Autodesk Inventor part; units mm, degrees
ref_plane "YZ Plane" through (0, 0, 0) normal (1, 0, 0) x (0, 1, 0)
ref_plane "XZ Plane" through (0, 0, 0) normal (0, 1, 0) x (-1, 0, 0)
ref_plane "XY Plane" through (0, 0, 0) normal (0, 0, 1) x (1, 0, 0)
sketch "Sketch2" plane through (0, 0, 0) normal (0, 0, 1) x (1, 0, 0)
  line L0 (0, 0) -> (76.2, 0)
  line L1 (76.2, 0) -> (76.2, 50.8)
  line L2 (76.2, 50.8) -> (0, 50.8)
  line L3 (0, 50.8) -> (0, 0)
  line L4 (-25.4, 0) -> (127, 0)
  line L5 (127, 0) -> (127, -50.8)
  line L6 (127, -50.8) -> (-25.4, -50.8)
  line L7 (-25.4, -50.8) -> (-25.4, 0)
  circle A0 centre (-19.05, -6.35) radius 3.175
  circle A1 centre (76.2, -44.45) radius 3.175
  line L8 (-17.8708, -3.4021) -> (77.3792, -41.5021)
  line L9 (-20.2292, -9.2979) -> (75.0208, -47.3979)
  circle A2 centre (25.4, -6.35) radius 3.175
  circle A3 centre (120.65, -44.45) radius 3.175
  line L10 (26.5792, -3.4021) -> (121.8292, -41.5021)
  line L11 (24.2208, -9.2979) -> (119.4708, -47.3979)
  dimension "d0" = 76.2
  dimension "d1" = 50.8
  dimension "d2" = 152.4
  dimension "d3" = 50.8
  dimension "d4" = 25.4
  dimension "d5" = 6.35
  dimension "d6" = 6.35
  dimension "d7" = 6.35
  dimension "d8" = 6.35
  dimension "d9" = 6.35
  dimension "d10" = 6.35
  dimension "d11" = 6.35
  dimension "d12" = 6.35
extrude "Extrusion1" add sketch "Sketch2" along normal blind 6.35
chamfer "Chamfer1" distance 6.35 angle 45 1 edges at (38.1, 50.8, 6.35)
properties part number "Short Wall Lift"
Here's how the part is built. I have some questions about the finished solid (model axes, mm). A direction names the side the tool comes from. Give positions to 0.01 mm unless a question says otherwise; leave off trailing zeros. Order: outer loops, then holes, each group sorted by start corner. A loop starts at its lowest first (then second) coordinate and runs counter-clockwise, first axis right, second up. Notation, with made-up numbers: M 31.25,12 L 78.25,12 A21 cw 78.25,37 Z; hole C 78.25,27.25 d4. An arc over 180 degrees is marked long. Answer as a JSON object with one key per item and string values. Group by question number.
1) We'd pull the mould along Y, two halves only. Please class faces 1 (the flat face through (52, -50.8, 3)), 2 (the flat face through (73.537, -22.185, 3.131)), 3 (the flat face through (127, -25, 3)), 4 (the cylindrical face through (123.623, -45.564, 3.131)): pulls with the +Y half, pulls with the -Y half, needs draft (parallel to the pull), parting line crosses it, or undercut.
2) On a 3-axis mill with a long thin cutter (end or side, diameter ignored), from which of +Z, -Z, +X, -X, +Y, -Y can I reach the whole of each face in a straight line? I mean faces 5 (the flat face through (37.6, 47.6, 3.2)), 6 (the flat face through (101, 0, 3)), 7 (the flat face through (29.087, -22.185, 3.131)), 8 (the flat face through (0, 26, 3)), 9 (the flat face through (50, -11, 0)). Say none if no direction works.
3) Suppose I cut it at C-C, the plane z = 4.5. Count the separate pieces of the cut face and the enclosed holes in it, plus the area to 3 significant figures.
4) Please list where these lines run through material, in increasing order: L1, parallel to Y at x = 54.5, z = 2.5; L2, parallel to Y at x = 38, z = 5.75; L3, parallel to X at y = 8, z = 1.5. Write a range as [from, to].
5) Suppose I cut it at B-B, the plane y = -17. Write out the boundary of the cut face in (x, z), plus the area to 3 significant figures.
6) I'm going to push flat-ended pins straight in: pin 1 Ø3 at (x, z) = (77.5, 2.5) entering from +Y; pin 2 Ø8 at (x, y) = (9.5, 29.5) entering from -Z; pin 3 Ø3 at (y, z) = (21.5, 3) entering from +X. Where does each tip first touch, or does it pass through?
Results found:
{
 "1": {"face 1": "pulls with the -Y half", "face 2": "undercut", "face 3": "needs draft", "face 4": "undercut"},
 "2": {"face 5": "+Z, +X, -X, +Y", "face 6": "+Z, -Z, +X, +Y", "face 7": "+Z, -Z", "face 8": "+Z, -Z, -X, +Y", "face 9": "-Z, +X, -X, +Y, -Y"},
 "3": {"separate pieces": "1", "enclosed holes": "2", "area": "9,900 mm²"},
 "4": {"L1": "[-50.8, -39.19], [-32.35, -21.41], [-14.57, 48.3]", "L2": "[-50.8, -32.59], [-25.75, -14.81], [-7.97, 45.05]", "L3": "[0, 76.2]"},
 "5": {"outline": "M -25.4,0 L -0.97,0 L -0.97,6.35 L -25.4,6.35 Z; M 16.12,0 L 43.48,0 L 43.48,6.35 L 16.12,6.35 Z; M 60.57,0 L 127,0 L 127,6.35 L 60.57,6.35 Z", "area": "751 mm²"},
 "6": {"pin 1": "y = 49.05", "pin 2": "z = 0", "pin 3": "x = 76.2"}
}
